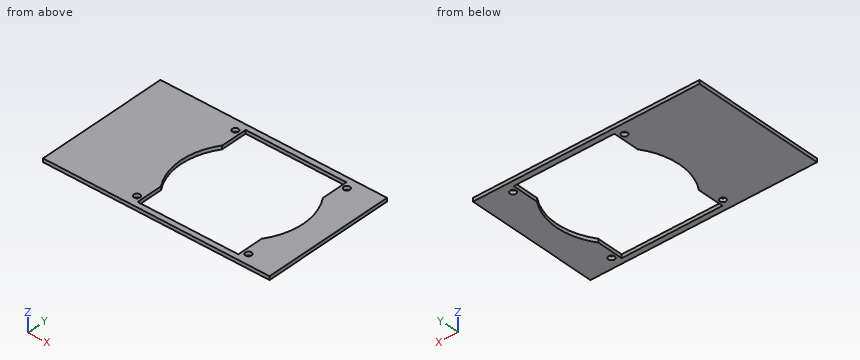
```python
from build123d import *

# Parameters (mm, degrees)
ESBO_O1_W                = 126
ESBO_O1_H                = 74
ESBO_O1_R                = 1.7
RESSALTO_EXTRUS_O1_DEPTH = 2


with BuildPart() as part:
    # Esboço1 → Ressalto-extrusão1 (new body)
    with BuildSketch(Plane.XY):
        with Locations((63, -37)):
            Rectangle(ESBO_O1_W, ESBO_O1_H)
        with Locations((47, -6)):
            Circle(ESBO_O1_R, mode=Mode.SUBTRACT)
        with Locations((109, -6)):
            Circle(ESBO_O1_R, mode=Mode.SUBTRACT)
        with Locations((47, -68)):
            Circle(ESBO_O1_R, mode=Mode.SUBTRACT)
        with Locations((109, -68)):
            Circle(ESBO_O1_R, mode=Mode.SUBTRACT)
        with BuildLine():
            Line((50, -3), (50, -17.712698478))
            ThreePointArc((50, -17.712698478), (44, -37), (50, -56.287301522))
            Line((50, -56.287301522), (50, -71))
            Line((50, -71), (106, -71))
            Line((106, -71), (106, -56.287301522))
            ThreePointArc((106, -56.287301522), (112, -37), (106, -17.712698478))
            Line((106, -17.712698478), (106, -3))
            Line((106, -3), (50, -3))
        make_face(mode=Mode.SUBTRACT)
    extrude(amount=RESSALTO_EXTRUS_O1_DEPTH)


solid = part.part
```
Check sheet for the modelled part. Datum: model origin and axes. Units: mm. Give positions to 0.01 mm unless a question says otherwise; leave off trailing zeros. Write each loop counter-clockwise with the first axis right and the second up, starting at its lowest first coordinate (ties: lowest second). Pieces come first, ordered by that corner, then holes. Notation, with made-up numbers: (-12.5, 62.5) -> (15.5, 62.5) arc R18 ccw to (15.5, 74.5) -> close; hole circle Ø9 at (-14.5, 79.5). An arc over 180 degrees is marked (long way). Use CSV: the item, a comma, the result in double quotes. Start each with the question number.
Q1. Cross-section at B-B on y = -6. Enter the section's corners in (x, z).
Q2. Cross-section at A-A on x = 63. Enter the section's corners in (y, z), and give its area (3 significant figures).
Q3. Cross-section at D-D on y = -65. Enter the section's corners in (x, z), and give its area (3 significant figures).
Q4. Cross-section at C-C on z = 1.4. Enter the section's corners in (x, y).
Q5. Depth check by flat-ended pin: P1, Ø5.5, axis at x = 47, y = -6, coming from the -Z side. Enter the tip coordinate at first touch or a pass-through.
Q6. Scan lines: line 1 along X through (y, z) = (-68, 0.8); line 2 along X through (y, z) = (-70, 1.85); line 3 along Y through (x, z) = (88.5, 0.95). Record each from-to range of solid material in increasing order.
Working result:
1,outline,"(0, 0) -> (45.3, 0) -> (45.3, 2) -> (0, 2) -> close; (48.7, 0) -> (50, 0) -> (50, 2) -> (48.7, 2) -> close; (106, 0) -> (107.3, 0) -> (107.3, 2) -> (106, 2) -> close; (110.7, 0) -> (126, 0) -> (126, 2) -> (110.7, 2) -> close"
2,outline,"(-74, 0) -> (-71, 0) -> (-71, 2) -> (-74, 2) -> close; (-3, 0) -> (0, 0) -> (0, 2) -> (-3, 2) -> close"
2,area,"12.0 mm^2"
3,outline,"(0, 0) -> (50, 0) -> (50, 2) -> (0, 2) -> close; (106, 0) -> (126, 0) -> (126, 2) -> (106, 2) -> close"
3,area,"140 mm^2"
4,outline,"(0, -74) -> (126, -74) -> (126, 0) -> (0, 0) -> close; hole circle Ø3.4 at (47, -68); hole circle Ø3.4 at (47, -6); hole (50, -71) -> (106, -71) -> (106, -56.29) arc R34 ccw to (106, -17.71) -> (106, -3) -> (50, -3) -> (50, -17.71) arc R34 ccw to (50, -56.29) -> close; hole circle Ø3.4 at (109, -68); hole circle Ø3.4 at (109, -6)"
5,P1,"stops at z = 0"
6,line 1,"x = 0 to 45.3, 48.7 to 50, 106 to 107.3, 110.7 to 126"
6,line 2,"x = 0 to 50, 106 to 126"
6,line 3,"y = -74 to -71, -3 to 0"
